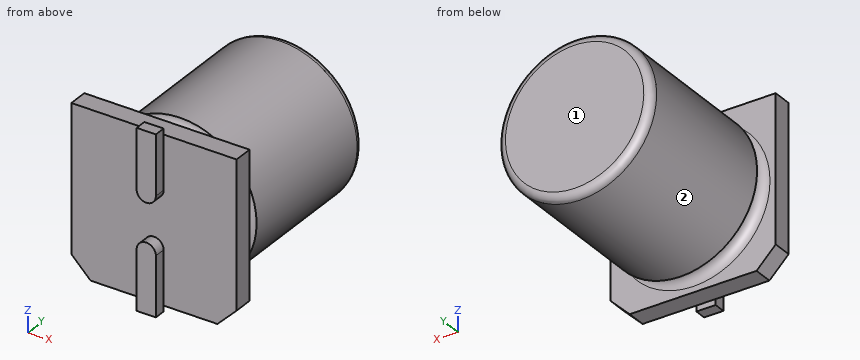
from build123d import *

# Parameters (mm, degrees)
BOSS_EXTRUDE1_DEPTH   = 0.3
BOSS_EXTRUDE1_2_DEPTH = 0.3
BOSS_EXTRUDE2_DEPTH   = 0.5
SKETCH4_R             = 2
BOSS_EXTRUDE3_DEPTH   = 4.6
FILLET1_R             = 0.2
SKETCH6_R             = 0.25


with BuildPart() as part:
    # Sketch1 → Boss-Extrude1 (new body)
    with BuildSketch(Plane(origin=(0, 0, 0), x_dir=(1, 0, 0), z_dir=(0, 1, 0))):
        with BuildLine():
            Line((0.25, 0.75), (0.25, 2.3))
            Line((0.25, 2.3), (-0.25, 2.3))
            Line((-0.25, 2.3), (-0.25, 0.75))
            ThreePointArc((-0.25, 0.75), (0, 0.5), (0.25, 0.75))
        make_face()
    extrude(amount=BOSS_EXTRUDE1_DEPTH)



with BuildPart() as body_2:
    # Sketch1 → Boss-Extrude1 2 (new body)
    with BuildSketch(Plane(origin=(0, 0, 0), x_dir=(1, 0, 0), z_dir=(0, 1, 0))):
        with BuildLine():
            Line((0.25, -0.75), (0.25, -2.3))
            Line((0.25, -2.3), (-0.25, -2.3))
            Line((-0.25, -2.3), (-0.25, -0.75))
            ThreePointArc((-0.25, -0.75), (0, -0.5), (0.25, -0.75))
        make_face()
    extrude(amount=BOSS_EXTRUDE1_2_DEPTH)


with BuildPart() as part_1:
    add(part.part)

    add(body_2.part)  # Boss-Extrude2 merges body 2
    # Sketch3 → Boss-Extrude2 (add)
    with BuildSketch(Plane(origin=(0, 0.3, 0), x_dir=(1, 0, 0), z_dir=(0, 1, 0))):
        Polygon((-2.15, -2.15), (2.15, -2.15), (2.15, 1.65), (1.65, 2.15), (-1.65, 2.15), (-2.15, 1.65), align=None)
    extrude(amount=BOSS_EXTRUDE2_DEPTH)

    # Sketch4 → Boss-Extrude3 (add)
    with BuildSketch(Plane(origin=(0, 0.8, 0), x_dir=(1, 0, 0), z_dir=(0, 1, 0))):
        with Locations(Location((0, 0, 0), (0, 0, 90))):
            Circle(SKETCH4_R)
    extrude(amount=BOSS_EXTRUDE3_DEPTH)

    # Fillet1
    fillet1_edges = [part_1.edges().sort_by_distance(p)[0] for p in [
        (0, 5.4, 2),
    ]]
    fillet(fillet1_edges, radius=FILLET1_R)

    # Sketch6 → Cut-Revolve1 (revolve, cut)
    with BuildSketch(Plane.XY, mode=Mode.PRIVATE) as cut_revolve1_sk:
        with Locations((2, 1.05)):
            Circle(SKETCH6_R)
    revolve(cut_revolve1_sk.sketch.rotate(Axis((0, 0, 0), (0, 1, 0)), 90), axis=Axis((0, 0, 0), (0, 1, 0)), mode=Mode.SUBTRACT)


solid = part_1.part
Read the model definition and answer for the solid it produces. Units are mm, in the model's axes. Face numbers are marked on the shaded views. A direction names the side the tool comes from. Give positions to 0.01 mm unless a question says otherwise; leave off trailing zeros. Loops run counter-clockwise (first coordinate to the right, second up) from the corner with the lowest first, then second, coordinate; pieces in that order, holes last. Notation, with made-up numbers: (77.5, 51.25) -> (102.5, 51.25) arc R20 cw to (102.5, 60.25) -> close; hole circle Ø2 at (81, 39). An arc over 180 degrees is marked (long way). Use a Markdown table: item, result.
Q1. Find the intervals of material crossed by line 1 along Z through (x, y) = (-0.7, 0.7); line 2 along Y through (x, z) = (-0.7, -0.3); line 3 along Y through (x, z) = (0.95, -1.85), in increasing order.
Solved:
| item | result |
|---|---|
| line 1 | z = -2.15 to 2.15 |
| line 2 | y = 0.3 to 5.4 |
| line 3 | y = 0.3 to 0.8 |
Q2. Section C-C, the plane y = 4.25 is taken. Determine the outline of the cut face in (x, z), then the cut area to 3 significant figures.
Solved:
| item | result |
|---|---|
| outline | circle Ø4 at (0, 0) |
| area | 12.6 mm^2 |
Q3. Section A-A, the plane x = 0 is taken. Determine the outline of the cut face in (y, z), then the cut area to 3 significant figures.
Solved:
| item | result |
|---|---|
| outline | (0, -2.3) -> (0.3, -2.3) -> (0.3, -2.15) -> (0.8, -2.15) -> (0.8, -2) arc R0.25 cw to (1.3, -2) -> (5.2, -2) arc R0.2 ccw to (5.4, -1.8) -> (5.4, 1.8) arc R0.2 ccw to (5.2, 2) -> (1.3, 2) arc R0.25 cw to (0.8, 2) -> (0.8, 2.15) -> (0.3, 2.15) -> (0.3, 2.3) -> (0, 2.3) -> (0, 0.5) -> (0.3, 0.5) -> (0.3, -0.5) -> (0, -0.5) -> close |
| area | 21.4 mm^2 |
Q4. A tool of negligible diameter and unlimited length cuts with its end or side. For the marked faces 1 and 2, from which of +Z, -Z, +X, -X, +Y, -Y can it reach the whole face along a straight path? Write none if from no direction.
Solved:
| item | result |
|---|---|
| face 1 | +Z, -Z, +X, -X, +Y |
| face 2 | +Y |
Q5. Section B-B, the plane z = 0 is taken. Determine the outline of the cut face in (x, y).
Solved:
| item | result |
|---|---|
| outline | (-2.15, 0.3) -> (2.15, 0.3) -> (2.15, 0.8) -> (2, 0.8) arc R0.25 cw to (2, 1.3) -> (2, 5.2) arc R0.2 ccw to (1.8, 5.4) -> (-1.8, 5.4) arc R0.2 ccw to (-2, 5.2) -> (-2, 1.3) arc R0.25 cw to (-2, 0.8) -> (-2.15, 0.8) -> close |
Q6. Each of these flat-tipped pins is pushed along its axis until it touches: pin 1 (2 mm diameter, centred on x = 0, z = 0.5, fed in from -Y); pin 2 (2 mm diameter, centred on x = 0, y = 3, fed in from -Z); pin 3 (2 mm diameter, centred on x = 0, y = 1.5, fed in from -Z); pin 4 (1 mm diameter, centred on x = 1, z = 0, fed in from -Y). Where does it stop, or does it pass through?
Solved:
| item | result |
|---|---|
| pin 1 | stops at y = 0 |
| pin 2 | stops at z = -2 |
| pin 3 | stops at z = -2.15 |
| pin 4 | stops at y = 0.3 |
